from build123d import *

# Parameters (mm, degrees)
SKETCH1_W           = 17.6
SKETCH1_H           = 12.3
BOSS_EXTRUDE1_DEPTH = 1.6
SKETCH2_W           = 2.75
SKETCH2_H           = 2.75
BOSS_EXTRUDE2_DEPTH = 2.6
SKETCH3_W           = 0.65
SKETCH3_H           = 0.65
BOSS_EXTRUDE3_DEPTH = 5.7


with BuildPart() as part:
    # Sketch1 → Boss-Extrude1 (new body)
    with BuildSketch(Plane(origin=(0, 0, 0), x_dir=(1, 0, 0), z_dir=(0, 1, 0))):
        Rectangle(SKETCH1_W, SKETCH1_H)
    extrude(amount=BOSS_EXTRUDE1_DEPTH)

    # Sketch2 → Boss-Extrude2 (add)
    with BuildSketch(Plane.XZ):
        with Locations((-7.475, 3.905)):
            Rectangle(SKETCH2_W, SKETCH2_H)
        with Locations((-7.475, -3.905)):
            Rectangle(SKETCH2_W, SKETCH2_H)
        with Locations((7.475, -3.905)):
            Rectangle(SKETCH2_W, SKETCH2_H)
        with Locations((7.475, 3.905)):
            Rectangle(SKETCH2_W, SKETCH2_H)
    extrude(amount=BOSS_EXTRUDE2_DEPTH)

    # Sketch3 → Boss-Extrude3 (add)
    with BuildSketch(Plane.XZ.offset(2.6)):
        with Locations((7.62, -3.81)):
            Rectangle(SKETCH3_W, SKETCH3_H)
        with Locations((7.62, 3.81)):
            Rectangle(SKETCH3_W, SKETCH3_H)
        with Locations((-7.62, -3.81)):
            Rectangle(SKETCH3_W, SKETCH3_H)
        with Locations((-7.62, 3.81)):
            Rectangle(SKETCH3_W, SKETCH3_H)
    extrude(amount=BOSS_EXTRUDE3_DEPTH)


solid = part.part
Model file for the job. Use its own axes, mm. A direction names the side the tool comes from. Give positions to 0.01 mm unless a question says otherwise; leave off trailing zeros. Loops run counter-clockwise (first coordinate to the right, second up) from the corner with the lowest first, then second, coordinate; pieces in that order, holes last.
1) Wall check: line 1 (Z direction, x = 6.5, y = -2); line 2 (Z direction, x = 7.75, y = -3.5) (3 decimals); line 3 (Y direction, x = 2.25, z = -4.25). Give the ranges that are in metal, low to high.
2) Saw through at C-C (y = -0.25). Write the cut outline in (x, z), plus the area to 4 significant figures.
3) Flat gauge pins, fed straight in: pin 1 Ø0.5 at (y, z) = (-6.5, -4) entering from +X (3 decimals); pin 2 Ø4 at (x, y) = (-6.5, -5.5) entering from +Z (3 decimals); pin 3 Ø3 at (x, z) = (7.5, -3) entering from -Y; pin 4 Ø4 at (x, z) = (1.5, -3) entering from -Y. Where does each tip first touch, or does it go through?
4) Saw through at A-A (y = -3). Write the cut outline in (x, z) (3 decimals).
5) Pull direction X, two halves, no side cores. Call faces 1 (the flat face through (8.85, -1, 4)), 2 (the flat face through (6.1, -1, -4)), 3 (the flat face through (-7, -1, 5.28)), 4 (the flat face through (-8.85, -1, -4)): +X half, -X half, draft (parallel to the pull), parting line (faces both ways), or undercut.
6) Tool access for faces 5 (the flat face through (7, -1, -2.53)), 6 (the flat face through (-6.1, -1, -4)), 7 (the flat face through (8.8, 1, 0)): list every direction of +Z, -Z, +X, -X, +Y, -Y with a clear straight run to the whole face (end or side of a thin tool).
7) Saw through at B-B (z = -2.75). Write the cut outline in (x, y), plus the area to 3 significant figures.
8) Saw through at D-D (x = -1.75). Write the cut outline in (y, z), plus the area to 3 significant figures.
Answer block:
1. line 1: z = -5.28 to -2.53, 2.53 to 5.28
1. line 2: z = -4.135 to -3.485, 3.485 to 4.135
1. line 3: y = 0 to 1.6
2. outline: (-8.85, -5.28) - (-6.1, -5.28) - (-6.1, -2.53) - (-8.85, -2.53) - close; (-8.85, 2.53) - (-6.1, 2.53) - (-6.1, 5.28) - (-8.85, 5.28) - close; (6.1, -5.28) - (8.85, -5.28) - (8.85, -2.53) - (6.1, -2.53) - close; (6.1, 2.53) - (8.85, 2.53) - (8.85, 5.28) - (6.1, 5.28) - close
2. area: 30.25 mm2
3. pin 1: stops at x = 7.945
3. pin 2: stops at z = 4.135
3. pin 3: stops at y = -8.3
3. pin 4: stops at y = 0
4. outline: (-7.945, -4.135) - (-7.295, -4.135) - (-7.295, -3.485) - (-7.945, -3.485) - close; (-7.945, 3.485) - (-7.295, 3.485) - (-7.295, 4.135) - (-7.945, 4.135) - close; (7.295, -4.135) - (7.945, -4.135) - (7.945, -3.485) - (7.295, -3.485) - close; (7.295, 3.485) - (7.945, 3.485) - (7.945, 4.135) - (7.295, 4.135) - close
5. face 1: +X half
5. face 2: undercut
5. face 3: draft
5. face 4: -X half
6. face 5: +X, -X, -Y
6. face 6: +Z, -Z, -Y
6. face 7: +Z, -Z, +X, +Y
7. outline: (-8.85, -2.6) - (-6.1, -2.6) - (-6.1, 0) - (6.1, 0) - (6.1, -2.6) - (8.85, -2.6) - (8.85, 0) - (8.8, 0) - (8.8, 1.6) - (-8.8, 1.6) - (-8.8, 0) - (-8.85, 0) - close
7. area: 42.5 mm2
8. outline: (0, -6.15) - (1.6, -6.15) - (1.6, 6.15) - (0, 6.15) - close
8. area: 19.7 mm2
